Geometry check sheet. Reference: the model listing, model coordinates, mm. Give positions to 0.01 mm unless a question says otherwise; leave off trailing zeros. Order: outer loops, then holes, each group sorted by start corner. A loop starts at its lowest first (then second) coordinate and runs counter-clockwise, first axis right, second up. Notation, with made-up numbers: M 14.5,42 L 59.5,42 A12 cw 59.5,50 Z; hole C -37,-16 d11. An arc over 180 degrees is marked long. Use CSV: the item, a comma, the result in double quotes. Start each with the question number.
from build123d import *

# Parameters (mm, degrees)
SKETCH_1_W      = 9
SKETCH_1_H      = 8
SKETCH_1_R      = 0.85
SKETCH_1_R_2    = 1.15
EXTRUDE_1_DEPTH = 1


with BuildPart() as part:
    # Эскиз1 → Бобышка-Вытянуть1 (new body)
    with BuildSketch(Plane(origin=(0, 0, 0), x_dir=(1, 0, 0), z_dir=(0, 1, 0))):
        with Locations((4.5, 4)):
            Rectangle(SKETCH_1_W, SKETCH_1_H)
        with Locations((1.5, 6.5)):
            Circle(SKETCH_1_R, mode=Mode.SUBTRACT)
        with Locations((7.5, 6.5)):
            Circle(SKETCH_1_R, mode=Mode.SUBTRACT)
        with Locations((3.6, 1.5)):
            Circle(SKETCH_1_R_2, mode=Mode.SUBTRACT)
    extrude(amount=EXTRUDE_1_DEPTH)


solid = part.part
(1) Sectioned sample at C-C on y = 0.35. Record the cut outline in (x, z), then the cut area to 3 significant figures.
(2) Draft check along Z on faces 1 (the face through (4.4, 0.5, 0)), 2 (the face through (4, 1, -4)), 3 (the face through (2.31, 0.49, -6.76)), 4 (the face through (8.285, 0.493, -6.174)). Enter one of: +Z half, -Z half, draft (parallel to the pull), parting line (faces both ways), or undercut.
(3) Go/stop test with a flat-tipped pin: P1, Ø1.4, axis at x = 7.5, z = -6.5, coming from the -Y side. Record where the tip stops, or that it passes through.
(4) Thickness scan on line 1 (X direction, y = 0.8, z = -6.5); line 2 (X direction, y = 0.45, z = -1.5); line 3 (Z direction, x = 7.5, y = 0.45). Record the ranges inside material, lowest first.
(5) Sectioned sample at D-D on z = -1.5. Record the cut outline in (x, y).
(6) Sectioned sample at A-A on x = 8.25. Record the cut outline in (y, z), then the cut area to 3 significant figures.
(7) Sectioned sample at B-B on z = -6.5. Record the cut outline in (x, y).
Responses:
1,outline,"M 0,-8 L 9,-8 L 9,0 L 0,0 Z; hole C 1.5,-6.5 d1.7; hole C 3.6,-1.5 d2.3; hole C 7.5,-6.5 d1.7"
1,area,"63.3 mm2"
2,face 1,"+Z half"
2,face 2,"draft"
2,face 3,"undercut"
2,face 4,"undercut"
3,P1,"through"
4,line 1,"0 to 0.65, 2.35 to 6.65, 8.35 to 9"
4,line 2,"0 to 2.45, 4.75 to 9"
4,line 3,"-8 to -7.35, -5.65 to 0"
5,outline,"M 0,0 L 2.45,0 L 2.45,1 L 0,1 Z; M 4.75,0 L 9,0 L 9,1 L 4.75,1 Z"
6,outline,"M 0,-8 L 1,-8 L 1,-6.9 L 0,-6.9 Z; M 0,-6.1 L 1,-6.1 L 1,0 L 0,0 Z"
6,area,"7.20 mm2"
7,outline,"M 0,0 L 0.65,0 L 0.65,1 L 0,1 Z; M 2.35,0 L 6.65,0 L 6.65,1 L 2.35,1 Z; M 8.35,0 L 9,0 L 9,1 L 8.35,1 Z"
